Autodesk Inventor part; units mm, degrees
ref_plane "YZ Plane" through (0, 0, 0) normal (1, 0, 0) x (0, 1, 0)
ref_plane "XZ Plane" through (0, 0, 0) normal (0, 1, 0) x (-1, 0, 0)
ref_plane "XY Plane" through (0, 0, 0) normal (0, 0, 1) x (1, 0, 0)
sketch "Skizze1" plane through (0, 0, 0) normal (0, 0, 1) x (1, 0, 0)
  line L0 (0, 0) -> (138, 0)
  line L1 (0, 0) -> (0, 16.5)
  line L2 (0, 16.5) -> (14, 16.5)
  line L3 (14, 16.5) -> (14, 10)
  line L4 (14, 10) -> (28, 10)
  line L5 (28, 10) -> (28, 15)
  line L6 (28, 15) -> (35.9017, 15)
  line L7 (35.9017, 15) -> (35.9017, 10)
  line L8 (35.9017, 10) -> (57.9017, 10)
  line L9 (57.9017, 10) -> (57.9017, 15)
  line L10 (57.9017, 15) -> (75.9017, 15)
  line L11 (75.9017, 15) -> (75.9017, 10)
  line L12 (75.9017, 10) -> (89.9017, 10)
  line L13 (89.9017, 10) -> (89.9017, 16.5)
  line L14 (89.9017, 16.5) -> (103.9017, 16.5)
  line L15 (103.9017, 16.5) -> (103.9017, 10)
  line L16 (103.9017, 10) -> (138, 10)
  line L17 (138, 10) -> (138, 0)
  point P0 (28, 12.5)
  point P1 (103.9017, 13.25)
  point P2 (89.9017, 13.25)
  dimension "d0" = 138
  dimension "d1" = 14
  dimension "d2" = 14
  dimension "d3" = 7.9017
  dimension "d4" = 22
  dimension "d5" = 14
  dimension "d6" = 14
  dimension "d7" = 18
  dimension "d8" = 33
  dimension "d9" = 20
  dimension "d10" = 30
revolve "Umdrehung1" add sketch "Skizze1" angle 360 about axis through (0, 0, 0) along (1, 0, 0)
properties part number "lehrerfreund" material "Stahl, galvanisiert"
Part model, mm, in its own coordinate system. A direction names the side the tool comes from. Coordinates: 2 decimals unless noted, no trailing zeros. Write each loop counter-clockwise with the first axis right and the second up, starting at its lowest first coordinate (ties: lowest second). Pieces come first, ordered by that corner, then holes.
Item 1: Probe line 1 (X direction, y = 12.5, z = 4.5); line 2 (Z direction, x = 85.5, y = 0); line 3 (Z direction, x = 14.5, y = 8). List the from-to ranges inside material, lowest first.
Item 2: Mould opens along X. For faces 1 (the face through (103.902, 0, -11)), 2 (the face through (57.902, 3, -10)), 3 (the face through (121.19, -2.17, -9.76)) say: released by +X, released by -X, zero draft, split by the parting line, or undercut.
Item 3: Slice it at A-A (z = -12). Write the cut outline in (x, y).
Item 4: Slice it at D-D (x = 100). Write the cut outline in (y, z), and give its area (3 significant figures).
Item 5: Pin check, flat tips, straight feed: pin 1 (12 mm diameter, centred on y = 3, z = -13, fed in from -X); pin 2 (2 mm diameter, centred on y = -12.5, z = -1.5, fed in from +X); pin 3 (5 mm diameter, centred on x = 54.5, y = 9.5, fed in from -Z); pin 4 (8 mm diameter, centred on x = 97, z = -7, fed in from +Y) (3 decimals). Stop position of each tip, or through.
Item 6: Which spindle directions (+Z, -Z, +X, -X, +Y, -Y) get a long thin tool onto all of the face, cutting with end or side? Do faces 4 (the face through (21.1, -2.17, -9.76)), 5 (the face through (138, 0, 0)). Say none if no direction does.
Results found:
1. line 1: x = 0 to 14, 28 to 35.9, 57.9 to 75.9, 89.9 to 103.9
1. line 2: z = -10 to 10
1. line 3: z = -6 to 6
2. face 1: released by +X
2. face 2: undercut
2. face 3: zero draft
3. outline: (0, -11.32) - (14, -11.32) - (14, 11.32) - (0, 11.32) - close; (28, -9) - (35.9, -9) - (35.9, 9) - (28, 9) - close; (57.9, -9) - (75.9, -9) - (75.9, 9) - (57.9, 9) - close; (89.9, -11.32) - (103.9, -11.32) - (103.9, 11.32) - (89.9, 11.32) - close
4. outline: circle Ø33 at (0, 0)
4. area: 855 mm2
5. pin 1: stops at x = 0
5. pin 2: stops at x = 103.9
5. pin 3: stops at z = -7.14
5. pin 4: stops at y = 16.225
6. face 4: none
6. face 5: +Z, -Z, +X, +Y, -Y
